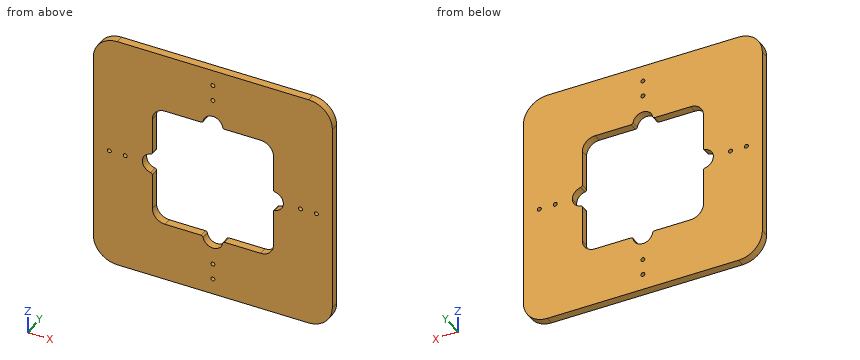
from build123d import *

# Parameters (mm, degrees)
BOSS_EXTRUDE3_DEPTH = 4
SKETCH2_R           = 2.5
BOSS_EXTRUDE4_DEPTH = 10
CUT_EXTRUDE1_DEPTH  = 52
CUT_EXTRUDE2_DEPTH  = 10


with BuildPart() as part:
    # Sketch1 → Boss-Extrude3 (new body)
    with BuildSketch(Plane(origin=(0, 0, 0), x_dir=(1, 0, 0), z_dir=(0, 1, 0))):
        with BuildLine():
            ThreePointArc((-75, -60), (-70.606601718, -70.606601718), (-60, -75))
            Line((-60, -75), (60, -75))
            ThreePointArc((60, -75), (70.606601718, -70.606601718), (75, -60))
            Line((75, -60), (75, 60))
            ThreePointArc((75, 60), (70.606601718, 70.606601718), (60, 75))
            Line((60, 75), (-60, 75))
            ThreePointArc((-60, 75), (-70.606601718, 70.606601718), (-75, 60))
            Line((-75, 60), (-75, -60))
        make_face()
    extrude(amount=BOSS_EXTRUDE3_DEPTH)

    # Sketch3 → Cut-Extrude1 (cut)
    with BuildSketch(Plane(origin=(0, 14, 0), x_dir=(1, 0, 0), z_dir=(0, 1, 0))):
        with BuildLine():
            Line((-60, 76), (60, 76))
            ThreePointArc((60, 76), (71.313708499, 71.313708499), (76, 60))
            Line((76, 60), (76, -60))
            ThreePointArc((76, -60), (71.313708499, -71.313708499), (60, -76))
            Line((60, -76), (-60, -76))
            ThreePointArc((-60, -76), (-71.313708499, -71.313708499), (-76, -60))
            Line((-76, -60), (-76, 60))
            ThreePointArc((-76, 60), (-71.313708499, 71.313708499), (-60, 76))
        make_face()
    extrude(amount=-CUT_EXTRUDE1_DEPTH, mode=Mode.SUBTRACT)


with BuildPart() as body_2:
    # Sketch2 → Boss-Extrude4 (new body)
    # profile 1 of 5: a face of its own
    with BuildSketch(Plane(origin=(0, 4, 0), x_dir=(1, 0, 0), z_dir=(0, 1, 0))):
        with BuildLine():
            ThreePointArc((150, -120), (141.213203436, -141.213203436), (120, -150))
            Line((120, -150), (-120, -150))
            ThreePointArc((-120, -150), (-141.213203436, -141.213203436), (-150, -120))
            Line((-150, -120), (-150, 120))
            ThreePointArc((-150, 120), (-141.213203436, 141.213203436), (-120, 150))
            Line((-120, 150), (120, 150))
            ThreePointArc((120, 150), (141.213203436, 141.213203436), (150, 120))
            Line((150, 120), (150, -120))
        make_face()
        with Locations(Location((-110, 0, 0), (0, 0, 270))):
            Circle(SKETCH2_R, mode=Mode.SUBTRACT)
        with Locations(Location((-130, 0, 0), (0, 0, 270))):
            Circle(SKETCH2_R, mode=Mode.SUBTRACT)
        with Locations(Location((130, 0, 0), (0, 0, 270))):
            Circle(SKETCH2_R, mode=Mode.SUBTRACT)
        with Locations(Location((110, 0, 0), (0, 0, 270))):
            Circle(SKETCH2_R, mode=Mode.SUBTRACT)
        with Locations(Location((0, -130, 0), (0, 0, 270))):
            Circle(SKETCH2_R, mode=Mode.SUBTRACT)
        with Locations(Location((0, -110, 0), (0, 0, 270))):
            Circle(SKETCH2_R, mode=Mode.SUBTRACT)
        with Locations(Location((0, 110, 0), (0, 0, 270))):
            Circle(SKETCH2_R, mode=Mode.SUBTRACT)
        with Locations(Location((0, 130, 0), (0, 0, 270))):
            Circle(SKETCH2_R, mode=Mode.SUBTRACT)
        Polygon((-76, -76), (-76, 76), (0, 76), (76, 76), (76, -76), align=None, mode=Mode.SUBTRACT)
    # profile 2 of 5: a face of its own
    with BuildSketch(Plane(origin=(0, 4, 0), x_dir=(1, 0, 0), z_dir=(0, 1, 0))):
        with BuildLine():
            ThreePointArc((-60, -76), (-71.313708499, -71.313708499), (-76, -60))
            Line((-76, -60), (-76, -76))
            Line((-76, -76), (-60, -76))
        make_face()
    # profile 3 of 5: a face of its own
    with BuildSketch(Plane(origin=(0, 4, 0), x_dir=(1, 0, 0), z_dir=(0, 1, 0))):
        with BuildLine():
            Line((76, -76), (76, -60))
            ThreePointArc((76, -60), (71.313708499, -71.313708499), (60, -76))
            Line((60, -76), (76, -76))
        make_face()
    # profile 4 of 5: a face of its own
    with BuildSketch(Plane(origin=(0, 4, 0), x_dir=(1, 0, 0), z_dir=(0, 1, 0))):
        with BuildLine():
            Line((76, 76), (60, 76))
            ThreePointArc((60, 76), (71.313708499, 71.313708499), (76, 60))
            Line((76, 60), (76, 76))
        make_face()
    # profile 5 of 5: a face of its own
    with BuildSketch(Plane(origin=(0, 4, 0), x_dir=(1, 0, 0), z_dir=(0, 1, 0))):
        with BuildLine():
            ThreePointArc((-76, 60), (-71.313708499, 71.313708499), (-60, 76))
            Line((-60, 76), (-76, 76))
            Line((-76, 76), (-76, 60))
        make_face()
    extrude(amount=BOSS_EXTRUDE4_DEPTH)

    # Sketch4 → Cut-Extrude2 (cut)
    with BuildSketch(Plane(origin=(0, 14, 0), x_dir=(1, 0, 0), z_dir=(0, 1, 0))):
        with BuildLine():
            Line((-12.5, 76), (12.5, 76))
            ThreePointArc((12.5, 76), (12.456214868, 77.045328257), (12.325166214, 78.08333334))
            ThreePointArc((12.325166214, 78.08333334), (-7.4e-08, 88.5), (-12.325166239, 78.083333193))
            ThreePointArc((-12.325166239, 78.083333193), (-12.456214874, 77.045328183), (-12.5, 76))
        make_face()
        with BuildLine():
            ThreePointArc((-12.5, 76), (0, 63.5), (12.5, 76))
            Line((12.5, 76), (-12.5, 76))
        make_face()
        with BuildLine():
            Line((-14.790199458, 76), (-12.5, 76))
            ThreePointArc((-12.5, 76), (-12.456214874, 77.045328183), (-12.325166239, 78.083333193))
            ThreePointArc((-12.325166239, 78.083333193), (-13.176456451, 76.590593415), (-14.790199458, 76))
        make_face()
        with BuildLine():
            ThreePointArc((12.325166214, 78.08333334), (12.456214868, 77.045328257), (12.5, 76))
            Line((12.5, 76), (14.790199431, 76))
            ThreePointArc((14.790199431, 76), (13.176456384, 76.590593471), (12.325166214, 78.08333334))
        make_face()
        with BuildLine():
            ThreePointArc((-76, -12.5), (-67.161165235, -8.838834765), (-63.5, 0))
            ThreePointArc((-63.5, 0), (-67.161165235, 8.838834765), (-76, 12.5))
            Line((-76, 12.5), (-76, -12.5))
        make_face()
        with BuildLine():
            Line((-76, -12.5), (-76, 12.5))
            ThreePointArc((-76, 12.5), (-77.045330875, 12.456214648), (-78.083338522, 12.325165338))
            ThreePointArc((-78.083338522, 12.325165338), (-88.5, -1.364e-06), (-78.083335831, -12.325165793))
            ThreePointArc((-78.083335831, -12.325165793), (-77.045329516, -12.456214762), (-76, -12.5))
        make_face()
        with BuildLine():
            ThreePointArc((-78.083338522, 12.325165338), (-77.045330875, 12.456214648), (-76, 12.5))
            Line((-76, 12.5), (-76, 14.790199458))
            ThreePointArc((-76, 14.790199458), (-76.590595159, 13.176454387), (-78.083338522, 12.325165338))
        make_face()
        with BuildLine():
            Line((-76, -14.790199458), (-76, -12.5))
            ThreePointArc((-76, -12.5), (-77.045329516, -12.456214762), (-78.083335831, -12.325165793))
            ThreePointArc((-78.083335831, -12.325165793), (-76.590594278, -13.17645543), (-76, -14.790199458))
        make_face()
        with BuildLine():
            Line((-12.5, -76), (12.5, -76))
            ThreePointArc((12.5, -76), (0, -63.5), (-12.5, -76))
        make_face()
        with BuildLine():
            ThreePointArc((12.325166095, -78.08333404), (12.456214838, -77.04532861), (12.5, -76))
            Line((12.5, -76), (-12.5, -76))
            ThreePointArc((-12.5, -76), (-12.456214619, -77.045331227), (-12.32516522, -78.083339217))
            ThreePointArc((-12.32516522, -78.083339217), (2.625e-06, -88.5), (12.325166095, -78.08333404))
        make_face()
        with BuildLine():
            ThreePointArc((-12.32516522, -78.083339217), (-12.456214619, -77.045331227), (-12.5, -76))
            Line((-12.5, -76), (-14.790199456, -76))
            ThreePointArc((-14.790199456, -76), (-13.176454117, -76.590595387), (-12.32516522, -78.083339217))
        make_face()
        with BuildLine():
            Line((14.790199458, -76), (12.5, -76))
            ThreePointArc((12.5, -76), (12.456214838, -77.04532861), (12.325166095, -78.08333404))
            ThreePointArc((12.325166095, -78.08333404), (13.176456123, -76.590593692), (14.790199458, -76))
        make_face()
        with BuildLine():
            ThreePointArc((78.083330118, -12.325166758), (85.547031645, -8.06871655), (88.5, 0))
            ThreePointArc((88.5, 0), (85.547032724, 8.068715273), (78.083333414, 12.325166201))
            ThreePointArc((78.083333414, 12.325166201), (77.045328294, 12.456214865), (76, 12.5))
            Line((76, 12.5), (76, -12.5))
            ThreePointArc((76, -12.5), (77.045326629, -12.456215005), (78.083330118, -12.325166758))
        make_face()
        with BuildLine():
            Line((76, -12.5), (76, 12.5))
            ThreePointArc((76, 12.5), (63.5, 0), (76, -12.5))
        make_face()
        with BuildLine():
            ThreePointArc((76, 12.5), (77.045328294, 12.456214865), (78.083333414, 12.325166201))
            ThreePointArc((78.083333414, 12.325166201), (76.590593423, 13.176456442), (76, 14.790199657))
            Line((76, 14.790199657), (76, 12.5))
        make_face()
        with BuildLine():
            ThreePointArc((76, -14.790199258), (76.590592472, -13.176457566), (78.083330118, -12.325166758))
            ThreePointArc((78.083330118, -12.325166758), (77.045326629, -12.456215005), (76, -12.5))
            Line((76, -12.5), (76, -14.790199258))
        make_face()
    extrude(amount=-CUT_EXTRUDE2_DEPTH, mode=Mode.SUBTRACT)


solid = body_2.part
For this review, take the finished solid that the model builds, in its own axes (mm). Round coordinates to 2 decimals unless told otherwise and drop trailing zeros. Order: outer loops, then holes, each group sorted by start corner. A loop starts at its lowest first (then second) coordinate and runs counter-clockwise, first axis right, second up. Notation, with made-up numbers: M 49,-35.75 L 90,-35.75 A21 ccw 90,-13.75 Z; hole C 26,-40 d9. An arc over 180 degrees is marked long. Write each question's results on one line, items separated by ' | '. Start each with the question number.
1. Clearance check with a flat-ended pin moving along its axis: pin 1 Ø3 at (x, z) = (0, -110) entering from -Y. State where the tip first meets the part, or that it passes through.
2. Add section A-A (x = -55.5). State the section outline as (y, z) points.
3. To check wall thickness, follow L1, parallel to Z at x = -37, y = 12.5; L2, parallel to X at y = 7.75, z = 110; L3, parallel to X at y = 9.25, z = -8.5. State the ranges of each line that lie inside material, in increasing order. Write a range as [from, to].
4. Add section C-C (y = 7.5). State how many separate pieces and enclosed holes the cut face has, then the cut area to 3 significant figures.
5. Add section B-B (z = 19). State the section outline as (x, y) points.
Output values:
1) pin 1: through
2) outline: M 4,-150 L 14,-150 L 14,-76 L 4,-76 Z; M 4,76 L 14,76 L 14,150 L 4,150 Z
3) L1: [-150, -76], [76, 150] | L2: [-150, -2.5], [2.5, 150] | L3: [-150, -85.17], [85.17, 150]
4) separate pieces: 1 | enclosed holes: 9 | area: 65,200 mm^2
5) outline: M -150,4 L -76,4 L -76,14 L -150,14 Z; M 76,4 L 150,4 L 150,14 L 76,14 Z
